from build123d import *

# Parameters (mm, degrees)
BOSS_EXTRUDE1_DEPTH      = 40
BOSS_EXTRUDE1_DEPTH_BACK = 40
SKETCH1_R                = 16
SKETCH2_W                = 50
SKETCH2_H                = 50
CUT_EXTRUDE1_DEPTH       = 151.416089565
SKETCH3_W                = 32
SKETCH3_H                = 50
CUT_EXTRUDE2_DEPTH       = 129.452325787
FILLET1_R                = 16
SKETCH4_W                = 29.06
SKETCH4_H                = 44.53
CUT_EXTRUDE3_DEPTH       = 133.382022949
FILLET2_R                = 14.53


with BuildPart() as part:
    # Sketch1 → Boss-Extrude1 (new, two sides: drawn at the far end of the back side and taken through both)
    with BuildSketch(Plane(origin=(0, 0, 0), x_dir=(0, 0, -1), z_dir=(1, 0, 0)).offset(-BOSS_EXTRUDE1_DEPTH_BACK)):
        Polygon((-105, 0), (-20, 0), (-20, 20), (20, 20), (20, 0), (35, 0), (35, 100), (-35, 100), (-35, 30), (-105, 30), align=None)
        with Locations((0, 70)):
            Circle(SKETCH1_R, mode=Mode.SUBTRACT)
    extrude(amount=BOSS_EXTRUDE1_DEPTH + BOSS_EXTRUDE1_DEPTH_BACK)

    # Sketch2 → Cut-Extrude1 (cut, through all)
    with BuildSketch(Plane(origin=(0, 100, 0), x_dir=(1, 0, 0), z_dir=(0, 1, 0))):
        Rectangle(SKETCH2_W, SKETCH2_H)
    extrude(amount=-CUT_EXTRUDE1_DEPTH, mode=Mode.SUBTRACT)

    # Sketch3 → Cut-Extrude2 (cut, through all)
    with BuildSketch(Plane.XY.offset(35)):
        with Locations((0, 75)):
            Rectangle(SKETCH3_W, SKETCH3_H)
    extrude(amount=-CUT_EXTRUDE2_DEPTH, mode=Mode.SUBTRACT)

    # Fillet1
    fillet1_edges = [part.edges().sort_by_distance(p)[0] for p in [
        (-16, 50, -30),
        (16, 50, -30),
        (16, 50, 30),
        (-16, 50, 30),
    ]]
    fillet(fillet1_edges, radius=FILLET1_R - 0.0001)  # a hair under: the kernel refuses the full size

    # Sketch4 → Cut-Extrude3 (cut, through all)
    with BuildSketch(Plane(origin=(0, 30, 0), x_dir=(1, 0, 0), z_dir=(0, 1, 0))):
        with Locations((0, -82.735)):
            Rectangle(SKETCH4_W, SKETCH4_H)
    extrude(amount=-CUT_EXTRUDE3_DEPTH, mode=Mode.SUBTRACT)

    # Fillet2
    fillet2_edges = [part.edges().sort_by_distance(p)[0] for p in [
        (14.53, 15, 60.47),
        (-14.53, 15, 60.47),
    ]]
    fillet(fillet2_edges, radius=FILLET2_R - 0.0001)  # a hair under: the kernel refuses the full size


solid = part.part
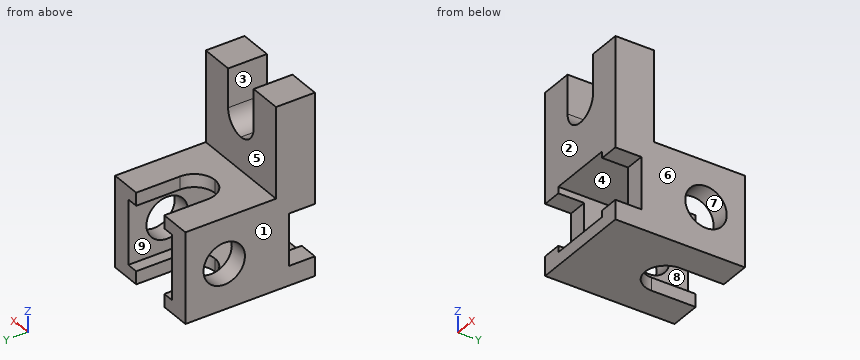
Source: CAD feature listing. Evaluate the final solid. Frame: model axes, mm. Face numbers are marked on the shaded views. A direction names the side the tool comes from. Give positions to 0.01 mm unless a question says otherwise; leave off trailing zeros. Order: outer loops, then holes, each group sorted by start corner. A loop starts at its lowest first (then second) coordinate and runs counter-clockwise, first axis right, second up. Notation, with made-up numbers: (35, 13) -> (61, 13) arc R12 cw to (61, 26) -> close; hole circle Ø7 at (48.25, 68.25). An arc over 180 degrees is marked (long way). Use a Markdown table: item, result.
1) Mould query, pull axis X, two halves, no side actions, for the marked faces 6, 7, 8 and 9. Classes: +X half, -X half, draft (parallel to the pull), parting line (faces both ways), or undercut.
Answer list:
| item | result |
|---|---|
| face 6 | +X half |
| face 7 | draft |
| face 8 | undercut |
| face 9 | undercut |
2) Reachability of the marked faces 1, 2, 3, 4 and 5 from +Z, -Z, +X, -X, +Y, -Y: full face, straight path, thin tool, end or side. Return the list, or none.
Answer list:
| item | result |
|---|---|
| face 1 | +Z, -Z, -X, +Y, -Y |
| face 2 | +Z, -Z, +X, -X, -Y |
| face 3 | +Z, +Y, -Y |
| face 4 | +Y, -Y |
| face 5 | +Z, +X, -X, +Y |
3) Ray query, line 1 along X through (y, z) = (89.5, -13.5); line 2 along Y through (x, z) = (-30, 0); line 3 along X through (y, z) = (87, -28). Return the intervals inside material, ascending. Write a range as [from, to].
Answer list:
| item | result |
|---|---|
| line 1 | [-40, -25], [25, 40] |
| line 2 | [20, 54], [86, 100] |
| line 3 | [-40, -16], [16, 40] |
4) Section query C-C, the plane z = 0. Return the cut outline in (x, y), then the cut area to 3 significant figures.
Answer list:
| item | result |
|---|---|
| outline | (-40, 20) -> (-25, 20) -> (-25, 54) -> (-40, 54) -> close; (-40, 86) -> (-25, 86) -> (-25, 100) -> (-40, 100) -> close; (25, 20) -> (40, 20) -> (40, 54) -> (25, 54) -> close; (25, 86) -> (40, 86) -> (40, 100) -> (25, 100) -> close |
| area | 1,440 mm² |
5) Section query B-B, the plane y = 70. Return the cut outline in (x, z).
Answer list:
| item | result |
|---|---|
| outline | (-40, -35) -> (-16, -35) -> (-16, -25) -> (-25, -25) -> (-25, -16) -> (-40, -16) -> close; (-40, 16) -> (-25, 16) -> (-25, 25) -> (-16, 25) -> (-16, 35) -> (-40, 35) -> close; (16, -35) -> (40, -35) -> (40, -16) -> (25, -16) -> (25, -25) -> (16, -25) -> close; (16, 25) -> (25, 25) -> (25, 16) -> (40, 16) -> (40, 35) -> (16, 35) -> close |
6) Contact query for flat-ended pins moving along their axis: P1, Ø21, axis at x = 9.5, z = 84, coming from the +Y side; P2, Ø3, axis at x = 21, y = 39.5, coming from the +Z side. Output: stop coordinate, or through.
Answer list:
| item | result |
|---|---|
| P1 | y = 30 |
| P2 | z = 35 |
7) Section query A-A, the plane x = -20.5. Return the cut outline in (y, z).
Answer list:
| item | result |
|---|---|
| outline | (0, -35) -> (100, -35) -> (100, -25) -> (0, -25) -> close; (0, 25) -> (100, 25) -> (100, 35) -> (30, 35) -> (30, 105) -> (0, 105) -> close |
8) Section query D-D, the plane y = 33. Return the cut outline in (x, z).
Answer list:
| item | result |
|---|---|
| outline | (-40, -35) -> (40, -35) -> (40, 35) -> (-40, 35) -> close; hole (-25, -25) -> (25, -25) -> (25, 25) -> (-25, 25) -> close |
